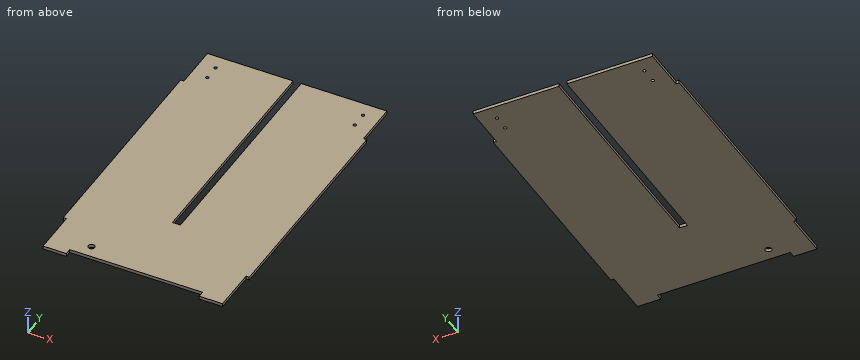
```python
from build123d import *

# Parameters (mm, degrees)
SKETCH2_W           = 3.175
SKETCH2_H           = 44.45
SKETCH2_W_2         = 23.132142857
SKETCH2_H_2         = 6.35
SKETCH2_W_3         = 26.307142857
BOSS_EXTRUDE1_DEPTH = 3.175
SKETCH3_W           = 7.9375
SKETCH3_H           = 228.6
CUT_EXTRUDE1_DEPTH  = 184.546857096
SKETCH4_R           = 3.175
CUT_EXTRUDE2_DEPTH  = 184.546857096
SKETCH5_R           = 1.5
CUT_EXTRUDE3_DEPTH  = 3.175
SKETCH6_W           = 3.175
SKETCH6_H           = 44.45
BOSS_EXTRUDE2_DEPTH = 3.175
SKETCH7_W           = 26.307142857
SKETCH7_H           = 6.35
CUT_EXTRUDE4_DEPTH  = 3.175


with BuildPart() as part:
    # Sketch2 → Boss-Extrude1 (new body)
    with BuildSketch(Plane.XY):
        Polygon((0, -152.4), (0, 152.4), (-88.9, 152.4), (-88.9, 107.95), (-88.9, 63.5), (-88.9, 19.05), (-88.9, -25.4), (-88.9, -69.85), (-88.9, -114.3), (-88.9, -152.4), (-65.767857143, -152.4), (-39.460714286, -152.4), (-13.153571429, -152.4), align=None)
        Polygon((88.9, 152.4), (0, 152.4), (0, -152.4), (13.153571429, -152.4), (39.460714286, -152.4), (65.767857143, -152.4), (88.9, -152.4), (88.9, -114.3), (88.9, -69.85), (88.9, -25.4), (88.9, 19.05), (88.9, 63.5), (88.9, 107.95), align=None)
        with Locations((-90.4875, 85.725)):
            Rectangle(SKETCH2_W, SKETCH2_H)
        with Locations((-90.4875, -3.175)):
            Rectangle(SKETCH2_W, SKETCH2_H)
        with Locations((-90.4875, -92.075)):
            Rectangle(SKETCH2_W, SKETCH2_H)
        with Locations((-77.333928571, -155.575)):
            Rectangle(SKETCH2_W_2, SKETCH2_H_2)
        with Locations((-26.307142858, -155.575)):
            Rectangle(SKETCH2_W_3, SKETCH2_H_2)
        with Locations((26.307142858, -155.575)):
            Rectangle(SKETCH2_W_3, SKETCH2_H_2)
        with Locations((90.4875, -92.075)):
            Rectangle(SKETCH2_W, SKETCH2_H)
        with Locations((90.4875, -3.175)):
            Rectangle(SKETCH2_W, SKETCH2_H)
        with Locations((90.4875, 85.725)):
            Rectangle(SKETCH2_W, SKETCH2_H)
        with Locations((77.333928571, -155.575)):
            Rectangle(SKETCH2_W_2, SKETCH2_H_2)
    extrude(amount=BOSS_EXTRUDE1_DEPTH)

    # Sketch3 → Cut-Extrude1 (cut, through all)
    with BuildSketch(Plane.XY.offset(3.175)):
        with Locations((0, 38.1)):
            Rectangle(SKETCH3_W, SKETCH3_H)
    extrude(amount=-CUT_EXTRUDE1_DEPTH, mode=Mode.SUBTRACT)

    # Sketch4 → Cut-Extrude2 (cut, through all)
    with BuildSketch(Plane.XY.offset(3.175)):
        with Locations((-50.8, -139.7)):
            Circle(SKETCH4_R)
    extrude(amount=-CUT_EXTRUDE2_DEPTH, mode=Mode.SUBTRACT)

    # Sketch5 → Cut-Extrude3 (cut)
    with BuildSketch(Plane.XY.offset(3.175)):
        with Locations((-73.025, 137.4)):
            Circle(SKETCH5_R)
        with Locations((-73.025, 121.65)):
            Circle(SKETCH5_R)
        with Locations((73.025, 121.65)):
            Circle(SKETCH5_R)
        with Locations((73.025, 137.4)):
            Circle(SKETCH5_R)
    extrude(amount=-CUT_EXTRUDE3_DEPTH, mode=Mode.SUBTRACT)

    # Sketch6 → Boss-Extrude2 (add)
    with BuildSketch(Plane.XY.offset(3.175)):
        with Locations((-90.4875, 41.275)):
            Rectangle(SKETCH6_W, SKETCH6_H)
        with Locations((-90.4875, -47.625)):
            Rectangle(SKETCH6_W, SKETCH6_H)
        with Locations((90.4875, 41.275)):
            Rectangle(SKETCH6_W, SKETCH6_H)
        with Locations((90.4875, -47.625)):
            Rectangle(SKETCH6_W, SKETCH6_H)
    extrude(amount=-BOSS_EXTRUDE2_DEPTH)

    # Sketch7 → Cut-Extrude4 (cut)
    with BuildSketch(Plane.XY.offset(3.175)):
        with Locations((-26.307142858, -155.575)):
            Rectangle(SKETCH7_W, SKETCH7_H)
        with Locations((26.307142858, -155.575)):
            Rectangle(SKETCH7_W, SKETCH7_H)
    extrude(amount=-CUT_EXTRUDE4_DEPTH, mode=Mode.SUBTRACT)


solid = part.part
```
CAD build for the part. Positions are in the model's coordinates, mm. Round coordinates to 2 decimals unless told otherwise and drop trailing zeros. Write each loop counter-clockwise with the first axis right and the second up, starting at its lowest first coordinate (ties: lowest second). Pieces come first, ordered by that corner, then holes. Notation, with made-up numbers: (-38, -38) -> (-12, -38) arc R33 cw to (-12, -3) -> close; hole circle Ø11 at (71, 56.5). An arc over 180 degrees is marked (long way). Answer in a Markdown table with one row per item. Add a question column.
Item 1: Saw through at B-B, the plane x = -50.8. Write the cut outline in (y, z) (3 decimals).
Item 2: Saw through at C-C, the plane z = 1.45. Write the cut outline in (x, y) (3 decimals), then the cut area to 3 significant figures.
Item 3: Drop flat-ended pins along their axis: pin 1 Ø1 at (x, z) = (-90.5, 2) entering from -Y; pin 2 Ø1.8 at (x, y) = (-73.025, 137.4) entering from +Z; pin 3 Ø1.6 at (x, z) = (-90.5, 1.5) entering from +Y; pin 4 Ø1.5 at (x, z) = (-44.5, 2.5) entering from -Y. Give the stop position or say it passes through.
Item 4: Saw through at A-A, the plane y = -139.7. Write the cut outline in (x, z) (3 decimals), then the cut area to 3 significant figures.
Item 5: Drill centre lines: line 1 (X direction, y = 137.4, z = 1.5) (3 decimals); line 2 (X direction, y = -139.7, z = 2) (3 decimals); line 3 (X direction, y = 10, z = 1.05) (3 decimals). Where is each one in solid material? Low to high. Write a range as from..to.
Item 6: Saw through at D-D, the plane x = 20. Write the cut outline in (y, z) (3 decimals).
Findings below:
| question | item | result |
|---|---|---|
| 1 | outline | (-152.4, 0) -> (-142.875, 0) -> (-142.875, 3.175) -> (-152.4, 3.175) -> close; (-136.525, 0) -> (152.4, 0) -> (152.4, 3.175) -> (-136.525, 3.175) -> close |
| 2 | outline | (-92.075, -114.3) -> (-88.9, -114.3) -> (-88.9, -158.75) -> (-65.768, -158.75) -> (-65.768, -152.4) -> (65.768, -152.4) -> (65.768, -158.75) -> (88.9, -158.75) -> (88.9, -114.3) -> (92.075, -114.3) -> (92.075, 107.95) -> (88.9, 107.95) -> (88.9, 152.4) -> (3.969, 152.4) -> (3.969, -76.2) -> (-3.969, -76.2) -> (-3.969, 152.4) -> (-88.9, 152.4) -> (-88.9, 107.95) -> (-92.075, 107.95) -> close; hole circle Ø3 at (-73.025, 121.65); hole circle Ø3 at (-73.025, 137.4); hole circle Ø6.35 at (-50.8, -139.7); hole circle Ø3 at (73.025, 121.65); hole circle Ø3 at (73.025, 137.4) |
| 2 | area | 54,000 mm^2 |
| 3 | pin 1 | stops at y = -114.3 |
| 3 | pin 2 | passes through |
| 3 | pin 3 | stops at y = 107.95 |
| 3 | pin 4 | stops at y = -152.4 |
| 4 | outline | (-88.9, 0) -> (-53.975, 0) -> (-53.975, 3.175) -> (-88.9, 3.175) -> close; (-47.625, 0) -> (88.9, 0) -> (88.9, 3.175) -> (-47.625, 3.175) -> close |
| 4 | area | 544 mm^2 |
| 5 | line 1 | x = -88.9..-74.525, -71.525..-3.969, 3.969..71.525, 74.525..88.9 |
| 5 | line 2 | x = -88.9..-53.975, -47.625..88.9 |
| 5 | line 3 | x = -92.075..-3.969, 3.969..92.075 |
| 6 | outline | (-152.4, 0) -> (152.4, 0) -> (152.4, 3.175) -> (-152.4, 3.175) -> close |
